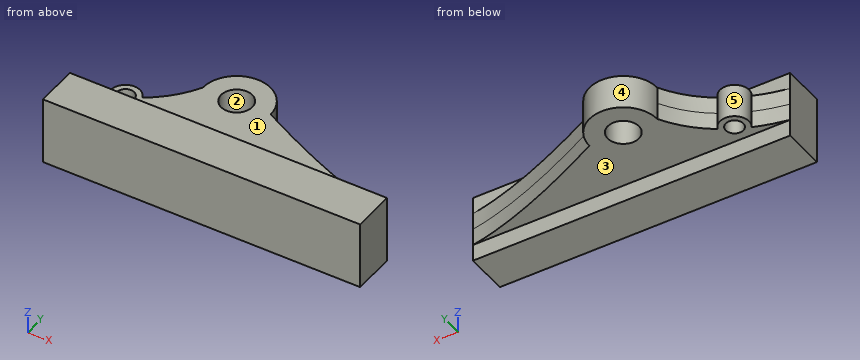
from build123d import *

# Parameters (mm, degrees)
SKETCH1_R               = 1.15
BOSS_EXTRUDE1_DEPTH     = 1.25
SKETCH2_W               = 23.360657125
SKETCH2_H               = 3.127548608
BOSS_EXTRUDE2_DEPTH     = 2.5
SKETCH3_R               = 1.070838979
BOSS_EXTRUDE3_DEPTH     = 2.5
CUT_EXTRUDE1_DEPTH      = 17.966509656
CUT_EXTRUDE1_DEPTH_BACK = 17.966509656
SKETCH4_R               = 0.65


with BuildPart() as part:
    # Sketch1 → Boss-Extrude1 (new, symmetric)
    with BuildSketch(Plane.XY):
        with BuildLine():
            Line((-10.268002202, 0), (13.092654923, 0))
            Line((13.092654923, 0), (13.092654923, 3.127548608))
            add(Edge.make_bspline(
                [(1.686549766, 7.618415505), (8.886011908, 3.875396255), (13.092654923, 3.127548608)],
                knots=[0, 0, 0, 1, 1, 1], degree=2))
            ThreePointArc((1.686549766, 7.618415505), (-0.813450234, 10.118415505), (-3.313450234, 7.618415505))
            add(Edge.make_bspline(
                [(-10.268002202, 3.127548608), (-5.306289346, 4.030602712), (-3.313450234, 7.618415505)],
                knots=[0, 0, 0, 1, 1, 1], degree=2))
            Line((-10.268002202, 3.127548608), (-10.268002202, 0))
        make_face()
        with Locations((-0.813450234, 7.618415505)):
            Circle(SKETCH1_R, mode=Mode.SUBTRACT)
    extrude(amount=BOSS_EXTRUDE1_DEPTH, both=True)

    # Sketch2 → Boss-Extrude2 (add, symmetric)
    with BuildSketch(Plane.XY):
        with Locations((1.412326361, 1.563774304)):
            Rectangle(SKETCH2_W, SKETCH2_H)
    extrude(amount=BOSS_EXTRUDE2_DEPTH, both=True)

    # Sketch3 → Boss-Extrude3 (add)
    with BuildSketch(Plane(origin=(0, 0, -1.25), x_dir=(-1, 0, 0), z_dir=(0, 0, -1))):
        with Locations((6.96167169, 4.380964726)):
            Circle(SKETCH3_R)
    extrude(amount=-BOSS_EXTRUDE3_DEPTH)

    # Sketch4 → Cut-Extrude1 (cut, two sides: drawn at the far end of the back side and taken through both)
    with BuildSketch(Plane(origin=(0, 0, -1.25), x_dir=(-1, 0, 0), z_dir=(0, 0, -1)).offset(-CUT_EXTRUDE1_DEPTH_BACK)):
        with Locations((6.96167169, 4.380964726)):
            Circle(SKETCH4_R)
    extrude(amount=CUT_EXTRUDE1_DEPTH + CUT_EXTRUDE1_DEPTH_BACK, mode=Mode.SUBTRACT)


with BuildPart() as part_1:
    # Body-Move/Copy1: moved
    add(part.part.moved(Location((0.81, -7.62, 0))))


solid = part_1.part
Could you check a few things on this model? Use its own coordinates, in mm. Face numbers are marked on the shaded views. A direction names the side the tool comes from. Round coordinates to 2 decimals unless told otherwise and drop trailing zeros. Write each loop counter-clockwise with the first axis right and the second up, starting at its lowest first coordinate (ties: lowest second). Pieces come first, ordered by that corner, then holes. Notation, with made-up numbers: (45, 16.25) - (59, 16.25) arc R27 cw to (59, 34.25) - close; hole circle Ø6 at (-10, -33.75). An arc over 180 degrees is marked (long way). Use a Markdown table: item, result.
Q1. Please list where these lines run through material, in increasing order: L1, parallel to Z at x = -1.5, y = 1.5; L2, parallel to Y at x = 0.5, z = 1.1; L3, parallel to Y at x = 10.75, z = -2.15.
Output values:
| item | result |
|---|---|
| L1 | -1.25 to 1.25 |
| L2 | -7.62 to -1.04, 1.03 to 2.45 |
| L3 | -7.62 to -4.49 |
Q2. Thinking about a two-plate mould opening in Y: for the marked faces 3, 4 and 5, which applies, released by +Y, released by -Y, zero draft, split by the parting line, or undercut?
Output values:
| item | result |
|---|---|
| face 3 | zero draft |
| face 4 | released by +Y |
| face 5 | undercut |
Q3. I want a section at B-B (z = 1.7). List the corners of the cut face in (x, y) for me, plus the area to 3 significant figures.
Output values:
| item | result |
|---|---|
| outline | (-9.46, -7.62) - (13.9, -7.62) - (13.9, -4.49) - (-9.46, -4.49) - close |
| area | 73.1 mm2 |
Q4. I want a section at A-A (x = -1.75). List the corners of the cut face in (y, z) for me.
Output values:
| item | result |
|---|---|
| outline | (-7.62, -2.5) - (-4.49, -2.5) - (-4.49, -1.25) - (1.79, -1.25) - (1.79, 1.25) - (-4.49, 1.25) - (-4.49, 2.5) - (-7.62, 2.5) - close |
Q5. I want a section at C-C (z = 0.3). Count the separate pieces of the cut face and the enclosed holes in it, plus the area to 3 significant figures.
Output values:
| item | result |
|---|---|
| separate pieces | 1 |
| enclosed holes | 2 |
| area | 134 mm2 |
Q6. For pin 1 (3 mm diameter, centred on y = -0.5, z = -1, fed in from +X); pin 2 (3.5 mm diameter, centred on x = 6.5, y = -1, fed in from -Z); pin 3 (0.6 mm diameter, centred on x = 1, z = 2, fed in from +Y); pin 4 (5 mm diameter, centred on x = 1.5, y = -2.5, fed in from +Z), each with a flat end and sliding along its axis, tell me the tip position at first contact or that it passes through.
Output values:
| item | result |
|---|---|
| pin 1 | x = 6.6 |
| pin 2 | z = -1.25 |
| pin 3 | y = -4.49 |
| pin 4 | z = 2.5 |
Q7. For the marked faces 1 and 2, which set-ups out of +Z, -Z, +X, -X, +Y, -Y let a thin tool reach every point of the face, with its end or its side?
Output values:
| item | result |
|---|---|
| face 1 | +Z, +X, -X, +Y |
| face 2 | +Z, -Z |
